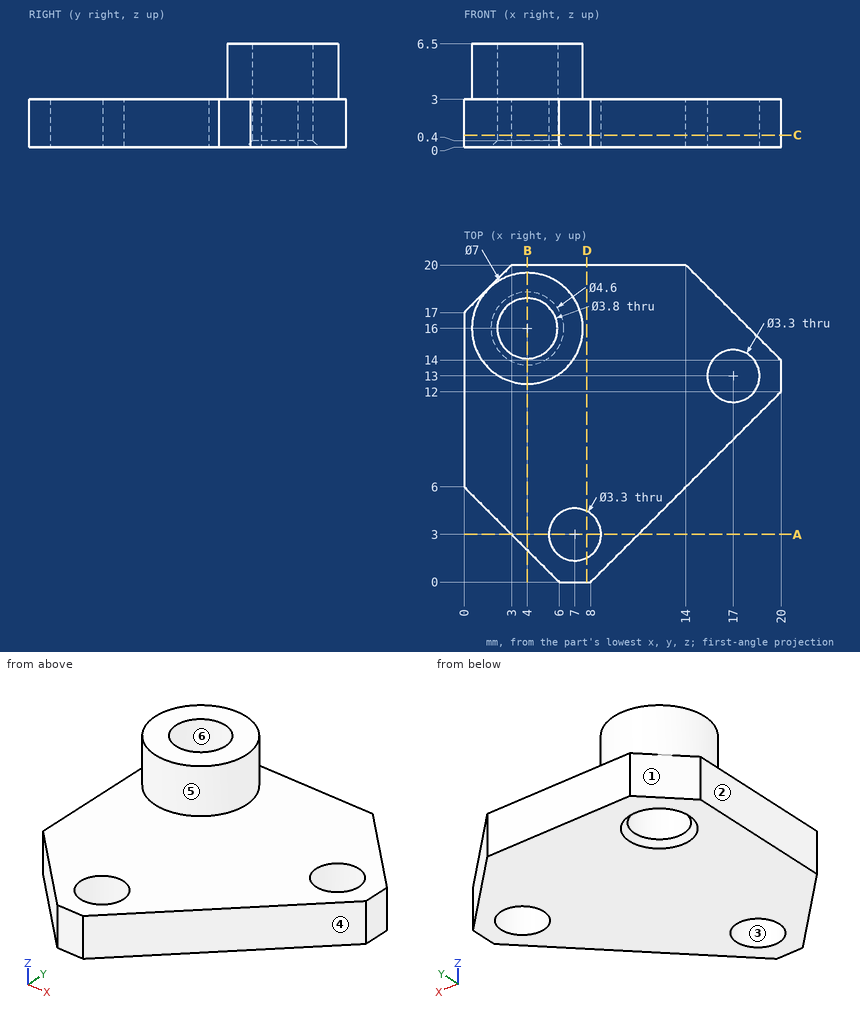
Study the drawing (mm; zero at the part's minimum x, y, z) and answer. A direction names the side the tool comes from. Round coordinates to 2 decimals unless told otherwise and drop trailing zeros. Write each loop counter-clockwise with the first axis right and the second up, starting at its lowest first coordinate (ties: lowest second). Pieces come first, ordered by that corner, then holes. Notation, with made-up numbers: (65.25, -37) - (71.25, -37) arc R10 ccw to (71.25, -22) - close; hole circle Ø5 at (36, 8.5). An arc over 180 degrees is marked (long way). Return JSON: item names as keys, results as strings. Group by question number.
Q1. Each of these flat-tipped pins is pushed along its axis until it touches: pin 1 Ø1.5 at (y, z) = (13.5, 3) entering from -X; pin 2 Ø1 at (y, z) = (6.5, 2.5) entering from +X; pin 3 Ø1.5 at (y, z) = (3, 3.5) entering from +X; pin 4 Ø4.5 at (x, y) = (17, 13) entering from +Z. Where does it stop, or does it pass through?
Q2. The part is cut by section A-A on y = 3. Write down the section's boundary in (x, z).
Q3. The part is cut by section C-C on z = 0.75. Write down the section's boundary in (x, y).
Q4. The mould has two halves that part along Y. Classify the marked faces 1, 2, 3 and 4: released by +Y, released by -Y, zero draft, split by the parting line, or undercut.
Q5. The part is cut by section D-D on x = 7.75. Write down the section's boundary in (y, z), then the cut area to 3 significant figures.
Q6. Find the intervals of material crossed by L1, parallel to Y at x = 7, z = 2.45; L2, parallel to Z at x = 11.5, y = 17.5; L3, parallel to Y at x = 11, z = 1.25, in increasing order.
Q7. For the marked faces 5 and 6, determine the directions among +Z, -Z, +X, -X, +Y, -Y from which every point of the face is accessible in a straight line to the end or side of a thin tool.
Q8. The part is cut by section B-B on x = 4. Write down the section's boundary in (y, z), then the cut area to 3 significant figures.
Solved:
{
 "1": {"pin 1": "x = 0", "pin 2": "x = 15", "pin 3": "x = 11.56", "pin 4": "z = 3"},
 "2": {"outline": "(3, 0) - (5.35, 0) - (5.35, 3) - (3, 3) - close; (8.65, 0) - (11, 0) - (11, 3) - (8.65, 3) - close"},
 "3": {"outline": "(0, 6) - (6, 0) - (8, 0) - (20, 12) - (20, 14) - (14, 20) - (3, 20) - (0, 17) - close; hole circle Ø3.8 at (4, 16); hole circle Ø3.3 at (7, 3); hole circle Ø3.3 at (17, 13)"},
 "4": {"face 1": "released by +Y", "face 2": "zero draft", "face 3": "undercut", "face 4": "released by -Y"},
 "5": {"outline": "(0, 0) - (1.53, 0) - (1.53, 3) - (0, 3) - close; (4.47, 0) - (20, 0) - (20, 3) - (4.47, 3) - close", "area": "51.2 mm²"},
 "6": {"L1": "0 to 1.35, 4.65 to 20", "L2": "0 to 3", "L3": "3 to 20"},
 "7": {"face 5": "+Z", "face 6": "+Z, -Z"},
 "8": {"outline": "(2, 0) - (13.7, 0) - (14.1, 0.4) - (14.1, 6.5) - (12.5, 6.5) - (12.5, 3) - (2, 3) - close; (17.9, 0.4) - (18.3, 0) - (20, 0) - (20, 3) - (19.5, 3) - (19.5, 6.5) - (17.9, 6.5) - close", "area": "53.6 mm²"}
}
